from build123d import *

# Parameters (mm, degrees)
SKETCH1_W               = 168
SKETCH1_H               = 141.165136176
BOSS_EXTRUDE1_DEPTH     = 90
CUT_EXTRUDE1_DEPTH      = 170.43110375
CUT_EXTRUDE1_DEPTH_BACK = 170.43110375


with BuildPart() as part:
    # Sketch1 → Boss-Extrude1 (new body)
    with BuildSketch(Plane(origin=(0, 0, 0), x_dir=(1, 0, 0), z_dir=(0, 1, 0))):
        with Locations((41, 0)):
            Rectangle(SKETCH1_W, SKETCH1_H)
    extrude(amount=BOSS_EXTRUDE1_DEPTH)

    # Sketch2 → Cut-Extrude1 (cut, two sides: drawn at the far end of the back side and taken through both)
    with BuildSketch(Plane.XY.offset(-CUT_EXTRUDE1_DEPTH_BACK)):
        Polygon((125, 90), (125, 10), (87, 10), (87, 55), (60, 55), (60, 90), align=None)
    extrude(amount=CUT_EXTRUDE1_DEPTH + CUT_EXTRUDE1_DEPTH_BACK, mode=Mode.SUBTRACT)


solid = part.part
Verification items for the finished model (mm, model axes). A direction names the side the tool comes from. Coordinates: 2 decimals unless noted, no trailing zeros. Order: outer loops, then holes, each group sorted by start corner. A loop starts at its lowest first (then second) coordinate and runs counter-clockwise, first axis right, second up. Notation, with made-up numbers: M -33,69.25 L 13,69.25 A13 cw 13,91.25 Z; hole C -8,56.5 d11. An arc over 180 degrees is marked long. One line per item, written item: value. Start each with the question number.
Item 1: Sectioned sample at C-C (y = 16). Enter the section's corners in (x, z), then the cut area to 3 significant figures.
Item 2: Gauge pin test, flat ends, axial feed: pin 1 (1.5 mm diameter, centred on x = 91.5, z = -36.5, fed in from +Y); pin 2 (4 mm diameter, centred on y = 21, z = 27.5, fed in from +X); pin 3 (10.5 mm diameter, centred on y = 73, z = -11.5, fed in from +X). Record the tip position at first contact, or that the pin passes through.
Item 3: Scan lines: probe 1 along X at (y, z) = (75, 34.5); probe 2 along X at (y, z) = (33.5, 47); probe 3 along Y at (x, z) = (104, -40). Record each from-to range of solid material in increasing order.
Item 4: Sectioned sample at A-A (z = 5.5). Enter the section's corners in (x, y).
Item 5: Access from +Z, -Z, +X, -X, +Y, -Y to the whole of each face (thin tool, end or side, straight path). Record for faces 1 (the flat face through (8, 90, -1)), 2 (the flat face through (87, 32, -1)).
Item 6: Sectioned sample at B-B (x = 98.5). Enter the section's corners in (y, z), then the cut area to 3 significant figures.
Conclusion:
1. outline: M -43,-70.58 L 87,-70.58 L 87,70.58 L -43,70.58 Z
1. area: 18,400 mm^2
2. pin 1: stops at y = 10
2. pin 2: stops at x = 87
2. pin 3: stops at x = 60
3. probe 1: x = -43 to 60
3. probe 2: x = -43 to 87
3. probe 3: y = 0 to 10
4. outline: M -43,0 L 125,0 L 125,10 L 87,10 L 87,55 L 60,55 L 60,90 L -43,90 Z
5. face 1: +Z, -Z, +X, -X, +Y
5. face 2: +Z, -Z, +X, +Y
6. outline: M 0,-70.58 L 10,-70.58 L 10,70.58 L 0,70.58 Z
6. area: 1,410 mm^2
